Autodesk Inventor part; units mm, degrees
ref_plane "YZ Plane" through (0, 0, 0) normal (1, 0, 0) x (0, 1, 0)
ref_plane "XZ Plane" through (0, 0, 0) normal (0, 1, 0) x (-1, 0, 0)
ref_plane "XY Plane" through (0, 0, 0) normal (0, 0, 1) x (1, 0, 0)
sketch "Sketch1" plane through (0, 0, 0) normal (1, 0, 0) x (0, 1, 0)
  arc A0 (19.5, 0) -> (-19.5, 0) centre (0, 0) ccw
  arc A1 (-19.5, -440) -> (19.5, -440) centre (0, -440) ccw
  line L0 (19.5, 0) -> (19.5, -440)
  line L1 (-19.5, 0) -> (-19.5, -440)
  dimension "d0" = 39
  dimension "d1" = 39
  dimension "d2" = 440
extrude "Extrusion1" add sketch "Sketch1" along normal blind 90
sketch "Sketch2" plane through (0, 0, 0) normal (-1, 0, 0) x (0, 0, 1)
  arc A0 (0, -19) -> (0, 19) centre (0, 0) ccw
  arc A1 (-440, 19.5) -> (-440, -19.5) centre (-440, 0) ccw
  arc A2 (-440, 19) -> (-440, -19) centre (-440, 0) ccw
  line L0 (-440, 19) -> (0, 19)
  line L1 (0, -19) -> (-440, -19)
  dimension "d5" = 38
  dimension "d6" = 38
extrude "Extrusion2" cut sketch "Sketch2" against normal through all
properties part number "Băng tải"
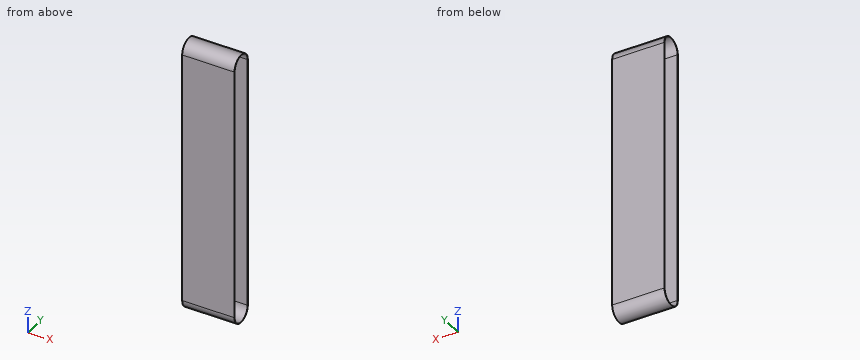
Verification items for the finished model (mm, model axes). Give positions to 0.01 mm unless a question says otherwise; leave off trailing zeros. Loops run counter-clockwise (first coordinate to the right, second up) from the corner with the lowest first, then second, coordinate; pieces in that order, holes last. Notation, with made-up numbers: (-34.5, -34) - (23.5, -34) arc R14 cw to (23.5, -22) - close; hole circle Ø7 at (23, 85). An arc over 180 degrees is marked (long way). Write item = value, one per line. Start each with the question number.
Q1. Cross-section at A-A, the plane z = -281.5. Enter the section's corners in (x, y).
Q2. Cross-section at B-B, the plane y = 0. Enter the section's corners in (x, z), and give its area (3 significant figures).
Q3. Thickness scan on line 1 (Y direction, x = 65, z = -384.5); line 2 (Z direction, x = 59.5, y = -1); line 3 (Z direction, x = 62, y = -2). Record the ranges inside material, lowest first.
Q4. Depth check by flat-ended pin: P1, Ø2, axis at x = 73.5, y = -8.5, coming from the +Z side; P2, Ø1.5, axis at x = 77.5, y = -13, coming from the -Z side; P3, Ø2, axis at x = 34.5, y = -7, coming from the +Z side. Enter the tip coordinate at first touch or a pass-through.
Q5. Cross-section at C-C, the plane x = 74. Enter the section's corners in (y, z).
Answer key:
q1.outline = (0, -19.5) - (90, -19.5) - (90, -19) - (0, -19) - close; (0, 19) - (90, 19) - (90, 19.5) - (0, 19.5) - close
q2.outline = (0, -459.5) - (90, -459.5) - (90, -459) - (0, -459) - close; (0, 19) - (90, 19) - (90, 19.5) - (0, 19.5) - close
q2.area = 90.0 mm^2
q3.line_1 = -19.5 to -19, 19 to 19.5
q3.line_2 = -459.47 to -458.97, 18.97 to 19.47
q3.line_3 = -459.4 to -458.89, 18.89 to 19.4
q4.P1 = 18
q4.P2 = -455.17
q4.P3 = 18.55
q5.outline = (-19.5, -440) arc R19.5 ccw to (19.5, -440) - (19.5, 0) arc R19.5 ccw to (-19.5, 0) - close; hole (-19, -440) arc R19 ccw to (19, -440) - (19, 0) arc R19 ccw to (-19, 0) - close
